```python
from build123d import *

# Parameters (mm, degrees)
F0_R     = 2.3
F0_R_2   = 0.5
F1_DEPTH = 22.75
F2_DEPTH = 4.25
F3_DEPTH = 7.25
F4_START = -4.5
F0_R_3   = 1
F4_DEPTH = 3.8
F5_START = -4.5
F0_W     = 5
F0_H     = 12.5
F5_DEPTH = 3.8
F6_DEPTH = 5.5


with BuildPart() as f1:
    # F0 (on Top) → F1 (new body)
    with BuildSketch(Plane.XY):
        Polygon((-11.5, -6.25), (11.5, -6.25), (11.5, 0), (11.5, 6.25), (-11.5, 6.25), align=None)
        with BuildLine():
            ThreePointArc((0.0380434783, 2.4833507514), (6.7704843308, 5.8639465861), (11.5, 0))
            ThreePointArc((11.5, 0), (6.7704843308, -5.8639465861), (0.0380434783, -2.4833507514))
            ThreePointArc((0.0380434783, -2.4833507514), (-2.75, 0), (0.0380434783, 2.4833507514))
        make_face(mode=Mode.SUBTRACT)
        with BuildLine():
            ThreePointArc((0.0380434783, -2.4833507514), (-0.5, 0), (0.0380434783, 2.4833507514))
            ThreePointArc((0.0380434783, 2.4833507514), (-2.75, 0), (0.0380434783, -2.4833507514))
        make_face()
        with BuildLine():
            ThreePointArc((2.25, 0), (1.6168300265, 1.6628125728), (0.0380434783, 2.4833507514))
            ThreePointArc((0.0380434783, 2.4833507514), (-0.5, 0), (0.0380434783, -2.4833507514))
            ThreePointArc((0.0380434783, -2.4833507514), (1.6168300265, -1.6628125728), (2.25, 0))
        make_face()
        with BuildLine():
            ThreePointArc((0.0380434783, -2.4833507514), (6.7704843308, -5.8639465861), (11.5, 0))
            ThreePointArc((11.5, 0), (6.7704843308, 5.8639465861), (0.0380434783, 2.4833507514))
            ThreePointArc((0.0380434783, 2.4833507514), (1.6168300265, 1.6628125728), (2.25, 0))
            ThreePointArc((2.25, 0), (1.6168300265, -1.6628125728), (0.0380434783, -2.4833507514))
        make_face()
        with Locations((5.5, 0)):
            Circle(F0_R, mode=Mode.SUBTRACT)
        with Locations((5.5, 0)):
            Circle(F0_R)
        with Locations((5.5, 0)):
            Circle(F0_R_2, mode=Mode.SUBTRACT)
    extrude(amount=-F1_DEPTH)

    # F0 (on Top) → F2 (join)
    with BuildSketch(Plane.XY):
        with BuildLine():
            ThreePointArc((0.0380434783, -2.4833507514), (6.7704843308, -5.8639465861), (11.5, 0))
            ThreePointArc((11.5, 0), (6.7704843308, 5.8639465861), (0.0380434783, 2.4833507514))
            ThreePointArc((0.0380434783, 2.4833507514), (1.6168300265, 1.6628125728), (2.25, 0))
            ThreePointArc((2.25, 0), (1.6168300265, -1.6628125728), (0.0380434783, -2.4833507514))
        make_face()
        with Locations((5.5, 0)):
            Circle(F0_R, mode=Mode.SUBTRACT)
        with Locations((5.5, 0)):
            Circle(F0_R)
        with Locations((5.5, 0)):
            Circle(F0_R_2, mode=Mode.SUBTRACT)
        with BuildLine():
            ThreePointArc((2.25, 0), (1.6168300265, 1.6628125728), (0.0380434783, 2.4833507514))
            ThreePointArc((0.0380434783, 2.4833507514), (-0.5, 0), (0.0380434783, -2.4833507514))
            ThreePointArc((0.0380434783, -2.4833507514), (1.6168300265, -1.6628125728), (2.25, 0))
        make_face()
        with BuildLine():
            ThreePointArc((0.0380434783, -2.4833507514), (-0.5, 0), (0.0380434783, 2.4833507514))
            ThreePointArc((0.0380434783, 2.4833507514), (-2.75, 0), (0.0380434783, -2.4833507514))
        make_face()
    extrude(amount=F2_DEPTH)

    # F0 (on Top) → F3 (join)
    with BuildSketch(Plane.XY):
        with Locations((5.5, 0)):
            Circle(F0_R)
        with Locations((5.5, 0)):
            Circle(F0_R_2, mode=Mode.SUBTRACT)
    extrude(amount=F3_DEPTH)

    # F0 (on Top) → F4 (join)
    with BuildSketch(Plane.XY.offset(F4_START)):
        Polygon((11.5, 0), (11.5, -6.25), (16.5, -6.25), (16.5, 6.25), (11.5, 6.25), align=None)
        with Locations((14, 0)):
            Circle(F0_R_3, mode=Mode.SUBTRACT)
    extrude(amount=-F4_DEPTH)

    # F0 (on Top) → F5 (join)
    with BuildSketch(Plane.XY.offset(F5_START)):
        with Locations((-14, 0)):
            Rectangle(F0_W, F0_H)
        with Locations((-14, 0)):
            Circle(F0_R_3, mode=Mode.SUBTRACT)
    extrude(amount=-F5_DEPTH)

    # F0 (on Top) → F6 (join)
    with BuildSketch(Plane.XY):
        with Locations((5.5, 0)):
            Circle(F0_R_2)
    extrude(amount=-F6_DEPTH)


solid = f1.part
```
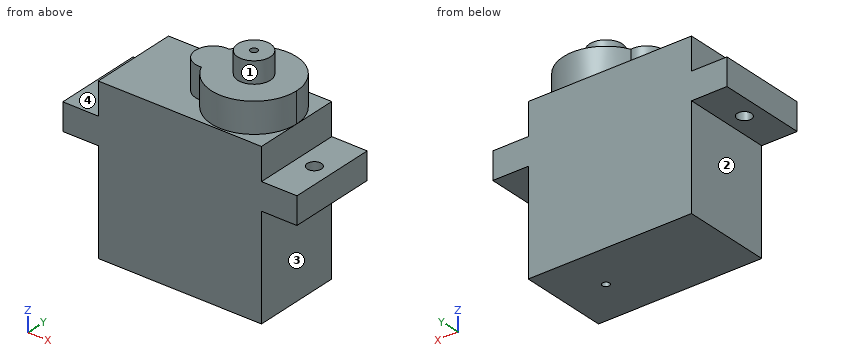
Source: CAD feature listing. Evaluate the final solid. Frame: model axes, mm. Face numbers are marked on the shaded views. A direction names the side the tool comes from. Give positions to 0.01 mm unless a question says otherwise; leave off trailing zeros. Loops run counter-clockwise (first coordinate to the right, second up) from the corner with the lowest first, then second, coordinate; pieces in that order, holes last. Notation, with made-up numbers: (53.25, 47.25) -> (92.25, 47.25) arc R18 cw to (92.25, 80.25) -> close; hole circle Ø1 at (85.5, -16.75). An arc over 180 degrees is marked (long way). Use a Markdown table: item, result. Add a question column.
(1) Section query C-C (x = 5.5). Output: boundary loops of the cut face in (y, z), then the cut area to 3 significant figures.
(2) Section query A-A (z = -7). Output: boundary loops of the cut face in (x, y), then the cut area to 3 significant figures.
(3) Access query for the marked faces 1, 2, 3 and 4. Directions: +Z, -Z, +X, -X, +Y, -Y. A direction counts if a zero-diameter tool reaches every point of the face in a straight line with its end or side. Return the directions, or none.
(4) Section query B-B (x = -14). Output: boundary loops of the cut face in (y, z).
(5) Section query D-D (y = 1.75). Output: boundary loops of the cut face in (x, z), then the cut area to 3 significant figures.
(6) First-contact query: pin 1 Ø3.5 at (y, z) = (-0.5, -2) entering from +X; pin 2 Ø1.5 at (x, y) = (13, 2.5) entering from +Z; pin 3 Ø3.5 at (y, z) = (-3, -1.5) entering from -X. Flat tips, straight axial feed; report the tip coordinate or a pass-through.
(7) Ray query, line 1 (Y direction, x = 5.5, z = -17.25); line 2 (Y direction, x = 14, z = -6.8); line 3 (Z direction, x = -13, y = -4.5). Return the intervals inside material, ascending.
Checked values:
| question | item | result |
|---|---|---|
| 1 | outline | (-6.25, -22.75) -> (-0.5, -22.75) -> (-0.5, -5.5) -> (0.5, -5.5) -> (0.5, -22.75) -> (6.25, -22.75) -> (6.25, 0) -> (6, 0) -> (6, 4.25) -> (2.3, 4.25) -> (2.3, 7.25) -> (0.5, 7.25) -> (0.5, 0) -> (-0.5, 0) -> (-0.5, 7.25) -> (-2.3, 7.25) -> (-2.3, 4.25) -> (-6, 4.25) -> (-6, 0) -> (-6.25, 0) -> close |
| 1 | area | 325 mm^2 |
| 2 | outline | (-16.5, -6.25) -> (16.5, -6.25) -> (16.5, 6.25) -> (-16.5, 6.25) -> close; hole circle Ø2 at (-14, 0); hole circle Ø1 at (5.5, 0); hole circle Ø2 at (14, 0) |
| 2 | area | 405 mm^2 |
| 3 | face 1 | +Z |
| 3 | face 2 | -Z, -X, +Y, -Y |
| 3 | face 3 | -Z, +X, +Y, -Y |
| 3 | face 4 | +Z, -X, +Y, -Y |
| 4 | outline | (-6.25, -8.3) -> (-1, -8.3) -> (-1, -4.5) -> (-6.25, -4.5) -> close; (1, -8.3) -> (6.25, -8.3) -> (6.25, -4.5) -> (1, -4.5) -> close |
| 5 | outline | (-16.5, -8.3) -> (-11.5, -8.3) -> (-11.5, -22.75) -> (11.5, -22.75) -> (11.5, -8.3) -> (16.5, -8.3) -> (16.5, -4.5) -> (11.5, -4.5) -> (11.5, 0) -> (11.24, 0) -> (11.24, 4.25) -> (6.99, 4.25) -> (6.99, 7.25) -> (4.01, 7.25) -> (4.01, 4.25) -> (-2.04, 4.25) -> (-2.04, 0) -> (-11.5, 0) -> (-11.5, -4.5) -> (-16.5, -4.5) -> close |
| 5 | area | 627 mm^2 |
| 6 | pin 1 | x = 11.5 |
| 6 | pin 2 | z = -4.5 |
| 6 | pin 3 | x = -11.5 |
| 7 | line 1 | -6.25 to -0.5, 0.5 to 6.25 |
| 7 | line 2 | -6.25 to -1, 1 to 6.25 |
| 7 | line 3 | -8.3 to -4.5 |
